The drawing under review shows one solid part. Ordinate dimensions are in mm from its lowest x, y, z. A direction names the side the tool comes from. Give positions to 0.01 mm unless a question says otherwise; leave off trailing zeros. Write item = value, one per line. Start each with the question number.
1. Mouldability with a two-part tool opening along X and no side actions: class the marked faces 1, 2 and 3 as pulls with the +X half, pulls with the -X half, needs draft (parallel to the pull), parting line crosses it, or undercut.
2. For P1, Ø3, axis at x = 2.5, z = 7.5, coming from the -Y side, flat-tipped, find the tip position at first contact; note if it passes through.
3. Machinability: for the marked faces 4 and 5, which of the approach directions +Z, -Z, +X, -X, +Y, -Y give a long, thin tool a straight path to every point of the face, cutting with its end or side? Answer none if there is none.
4. Wall thickness on probe 1 along X at (y, z) = (1.5, 17); probe 2 along Z at (x, y) = (6.25, 1) (1 decimal); probe 3 along Z at (x, y) = (6.5, 5) (1 decimal): over which ranges is each line inside the solid? List them lowest first.
5. We need section A-A, the plane y = 2. State how many separate pieces and enclosed holes the cut face has.
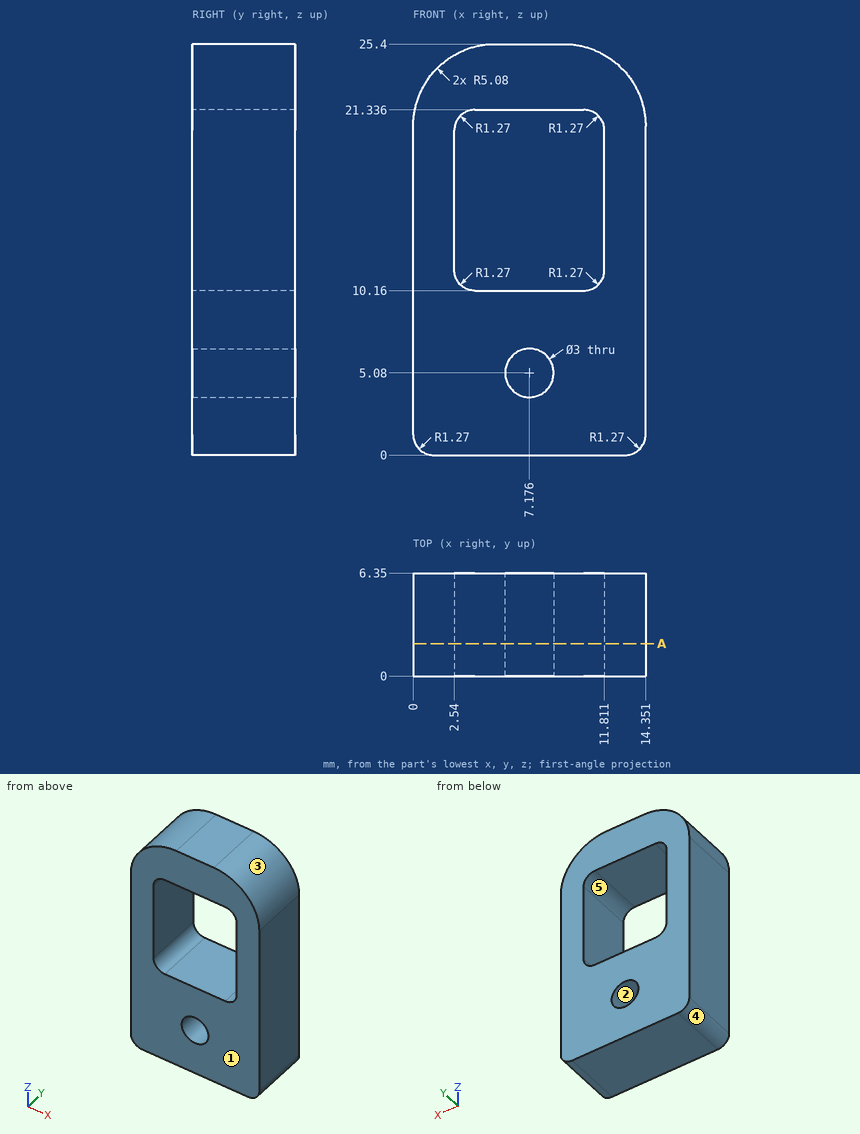
Model answer:
q1.face_1 = needs draft
q1.face_2 = undercut
q1.face_3 = pulls with the +X half
q2.P1 = 0
q3.face_4 = -Z, -X, +Y, -Y
q3.face_5 = +Y, -Y
q4.probe_1 = 0 to 2.54, 11.81 to 14.35
q4.probe_2 = 0 to 3.9, 6.3 to 10.2, 21.3 to 25.4
q4.probe_3 = 0 to 3.7, 6.4 to 10.2, 21.3 to 25.4
q5.separate_pieces = 1
q5.enclosed_holes = 2
